```python
from build123d import *

# Parameters (mm, degrees)
BOSS_EXTRUDE2_DEPTH  = 3.81
FILLET1_R            = 3.175
CUT_EXTRUDE1_REACH   = 61.178
SKETCH4_R            = 1.627
FILLET2_R            = 1.27
CUT_EXTRUDE2_REACH   = 60.809
SKETCH5_R            = 1.905
SKETCH6_W            = 38.1
SKETCH6_H            = 11.43
BOSS_EXTRUDE3_DEPTH  = 7.62
SKETCH7_R            = 2.54
BOSS_EXTRUDE4_DEPTH  = 8.89
SKETCH8_R            = 4.445
BOSS_EXTRUDE5_DEPTH  = 2
FILLET3_R            = 1.27
FILLET3_OF_MIRROR3_R = 1.27
FILLET4_R            = 0.635
CUT_EXTRUDE3_START   = -0.508
CUT_EXTRUDE3_DEPTH   = 0.508
SKETCH13_W           = 12.7
SKETCH13_H           = 3.81
CUT_EXTRUDE4_DEPTH   = 1.778
SKETCH14_W           = 11.811
SKETCH14_H           = 2.54
CUT_EXTRUDE5_DEPTH   = 2.54
SKETCH15_W           = 15.24
SKETCH15_H           = 6.35
BOSS_EXTRUDE6_DEPTH  = 1.778
BOSS_EXTRUDE7_DEPTH  = 2.54
BOSS_EXTRUDE8_DEPTH  = 2.54


# Read off the part's stored shape, not the designer's step: Cut-Extrude3
with BuildPart() as part:
    # Sketch3 → Boss-Extrude2 (new, symmetric)
    with BuildSketch(Plane.XY):
        Polygon((34.29, -3.175), (34.29, 3.175), (26.67, 3.175), (26.67, 41.275), (34.29, 41.275), (34.29, 47.625), (0, 47.625), (-34.29, 47.625), (-34.29, 41.275), (-26.67, 41.275), (-26.67, 3.175), (-34.29, 3.175), (-34.29, -3.175), (-19.05, -3.175), (-19.05, 0), (19.05, 0), (19.05, -3.175), align=None)
        Polygon((-19.05, 3.175), (-19.05, 41.275), (0, 41.275), (19.05, 41.275), (19.05, 3.175), align=None, mode=Mode.SUBTRACT)
    extrude(amount=BOSS_EXTRUDE2_DEPTH, both=True)

    # Fillet1
    fillet1_edges = [part.edges().sort_by_distance(p)[0] for p in [
        (34.29, 3.175, 0),
        (34.29, 41.275, 0),
        (34.29, 47.625, 0),
        (-34.29, 3.175, 0),
        (-34.29, 41.275, 0),
        (-34.29, 47.625, 0),
        (34.29, -3.175, 0),
        (-34.29, -3.175, 0),
    ]]
    fillet(fillet1_edges, radius=FILLET1_R - 0.0001)  # a hair under: the kernel refuses the full size

    # Sketch4 → Cut-Extrude1 (cut, up to next)
    with BuildSketch(Plane.XY.offset(3.81), mode=Mode.PRIVATE) as cut_extrude1_sk1:
        with Locations((-31.115, 44.45)):
            Circle(SKETCH4_R)
    cut_extrude1_tool1 = extrude(cut_extrude1_sk1.sketch, amount=-CUT_EXTRUDE1_REACH, mode=Mode.PRIVATE) & part.part
    # Sketch4 → Cut-Extrude1 (cut, up to next)
    with BuildSketch(Plane.XY.offset(3.81), mode=Mode.PRIVATE) as cut_extrude1_sk2:
        with Locations((-31.115, 0)):
            Circle(SKETCH4_R)
    cut_extrude1_tool2 = extrude(cut_extrude1_sk2.sketch, amount=-CUT_EXTRUDE1_REACH, mode=Mode.PRIVATE) & part.part
    cut_extrude1_1 = cut_extrude1_tool1.solids().sort_by_distance((-31.115, 44.45, 3.81))[0]
    add(cut_extrude1_1, mode=Mode.SUBTRACT)
    cut_extrude1_2 = cut_extrude1_tool2.solids().sort_by_distance((-31.115, 0, 3.81))[0]
    add(cut_extrude1_2, mode=Mode.SUBTRACT)
    cut_extrude1 = cut_extrude1_1 + cut_extrude1_2  # Cut-Extrude1 as one shape, for the pattern or mirror that repeats it

    # Mirror1: Cut-Extrude1 across plane
    add(cut_extrude1.mirror(Plane(origin=(0, 0, 0), x_dir=(0, 0, 1), z_dir=(1, 0, 0))), mode=Mode.SUBTRACT)

    # Fillet2
    fillet2_edges = [part.edges().sort_by_distance(p)[0] for p in [
        (-26.67, 22.225, -3.81),
        (26.67, 22.225, -3.81),
        (26.67, 22.225, 3.81),
        (-26.67, 22.225, 3.81),
    ]]
    fillet(fillet2_edges, radius=FILLET2_R)

    # Sketch5 → Cut-Extrude2 (cut, up to next)
    with BuildSketch(Plane.XZ, mode=Mode.PRIVATE) as cut_extrude2_sk1:
        with Locations((-15.24, 0)):
            Circle(SKETCH5_R)
    cut_extrude2_tool1 = extrude(cut_extrude2_sk1.sketch, amount=-CUT_EXTRUDE2_REACH, mode=Mode.PRIVATE) & part.part
    # Sketch5 → Cut-Extrude2 (cut, up to next)
    with BuildSketch(Plane.XZ, mode=Mode.PRIVATE) as cut_extrude2_sk2:
        with Locations(Location((15.24, 0, 0), (0, 0, 180))):
            Circle(SKETCH5_R)
    cut_extrude2_tool2 = extrude(cut_extrude2_sk2.sketch, amount=-CUT_EXTRUDE2_REACH, mode=Mode.PRIVATE) & part.part
    add(cut_extrude2_tool1.solids().sort_by_distance((-15.24, 0, 0))[0], mode=Mode.SUBTRACT)
    add(cut_extrude2_tool2.solids().sort_by_distance((15.24, 0, 0))[0], mode=Mode.SUBTRACT)

    # Sketch6 → Boss-Extrude3 (add)
    with BuildSketch(Plane.XY.offset(3.81)):
        with Locations((0, 11.1125)):
            Rectangle(SKETCH6_W, SKETCH6_H)
    extrude(amount=-BOSS_EXTRUDE3_DEPTH)

    # Sketch7 → Boss-Extrude4 (add)
    with BuildSketch(Plane.XY.offset(3.81)):
        with Locations(Location((-8.89, 11.176999998, 0), (0, 0, 180))):
            Circle(SKETCH7_R)
        with Locations(Location((8.89, 11.176999998, 0), (0, 0, 180))):
            Circle(SKETCH7_R)
    extrude(amount=BOSS_EXTRUDE4_DEPTH)

    # Sketch8 → Boss-Extrude5 (add)
    with BuildSketch(Plane.XY.offset(3.81)):
        with Locations(Location((-8.89, 11.176999998, 0), (0, 0, 180))):
            Circle(SKETCH8_R)
    boss_extrude5 = extrude(amount=BOSS_EXTRUDE5_DEPTH)

    # Fillet3
    fillet3_edges = [part.edges().sort_by_distance(p)[0] for p in [
        (-4.445, 11.176999998, 5.81),
    ]]
    fillet(fillet3_edges, radius=FILLET3_R)

    # Mirror3: Boss-Extrude5 across plane
    add(boss_extrude5.mirror(Plane(origin=(0, 0, 0), x_dir=(0, 0, 1), z_dir=(1, 0, 0))))

    # Fillet3 of Mirror3
    fillet3_of_mirror3_edges = [part.edges().sort_by_distance(p)[0] for p in [
        (4.445, 11.176999998, 5.81),
    ]]
    fillet(fillet3_of_mirror3_edges, radius=FILLET3_OF_MIRROR3_R)

    # Fillet4
    fillet4_edges = [part.edges().sort_by_distance(p)[0] for p in [
        (19.05, 4.28625, 3.81),
        (19.05, 4.28625, -3.81),
        (-19.05, 4.28625, 3.81),
        (-19.05, 4.28625, -3.81),
        (0, 16.8275, 3.81),
        (19.05, 3.175, 0),
        (-19.05, 3.175, 0),
        (0, 3.175, -3.81),
        (0, 3.175, 3.81),
    ]]
    fillet(fillet4_edges, radius=FILLET4_R)

    # Cut-Extrude3 outline → Cut-Extrude3 (cut)
    with BuildSketch(Plane(origin=(0, 0, -3.81), x_dir=(-1, 0, 0), z_dir=(0, 0, -1)).offset(CUT_EXTRUDE3_START)):
        Polygon((-36, 41.275), (-25.4, 41.275), (-25.4, 3.175), (-36, 3.175), (-36, -5), (36, -5), (36, 3.175), (25.4, 3.175), (25.4, 41.275), (36, 41.275), (36, 49), (-36, 49), align=None)
    extrude(amount=CUT_EXTRUDE3_DEPTH, mode=Mode.SUBTRACT)

    # Sketch13 → Cut-Extrude4 (cut)
    with BuildSketch(Plane.XY.offset(3.81)):
        with Locations((0, 43.18)):
            Rectangle(SKETCH13_W, SKETCH13_H)
    extrude(amount=-CUT_EXTRUDE4_DEPTH, mode=Mode.SUBTRACT)

    # Sketch14 → Cut-Extrude5 (cut)
    with BuildSketch(Plane(origin=(0, 0, -3.302), x_dir=(-1, 0, 0), z_dir=(0, 0, -1))):
        with Locations((0, 15.5575)):
            Rectangle(SKETCH14_W, SKETCH14_H)
    extrude(amount=-CUT_EXTRUDE5_DEPTH, mode=Mode.SUBTRACT)

    # Sketch15 → Boss-Extrude6 (add)
    with BuildSketch(Plane(origin=(0, 0, -3.302), x_dir=(-1, 0, 0), z_dir=(0, 0, -1))):
        with Locations((0, 44.45)):
            Rectangle(SKETCH15_W, SKETCH15_H)
        Polygon((-7.62, 16.8275), (-5.9055, 16.8275), (-5.9055, 14.2875), (5.9055, 14.2875), (5.9055, 16.8275), (7.62, 16.8275), (7.62, 9.2075), (-7.62, 9.2075), align=None)
    extrude(amount=BOSS_EXTRUDE6_DEPTH)

    # Sketch16 → Boss-Extrude7 (add)
    with BuildSketch(Plane(origin=(0, 0, -5.08), x_dir=(-1, 0, 0), z_dir=(0, 0, -1))):
        Polygon((-5.9055, 41.275), (-5.9055, 42.926), (5.9055, 42.926), (5.9055, 41.275), (7.62, 41.275), (7.62, 47.625), (-7.62, 47.625), (-7.62, 41.275), align=None)
    extrude(amount=BOSS_EXTRUDE7_DEPTH)

    # Sketch18 → Boss-Extrude8 (add)
    with BuildSketch(Plane(origin=(0, 0, -5.08), x_dir=(-1, 0, 0), z_dir=(0, 0, -1))):
        Polygon((-7.62, 16.8275), (-5.9055, 16.8275), (-5.9055, 10.4902), (5.9055, 10.4902), (5.9055, 16.8275), (7.62, 16.8275), (7.62, 9.2075), (-7.62, 9.2075), align=None)
    extrude(amount=BOSS_EXTRUDE8_DEPTH)


solid = part.part
```
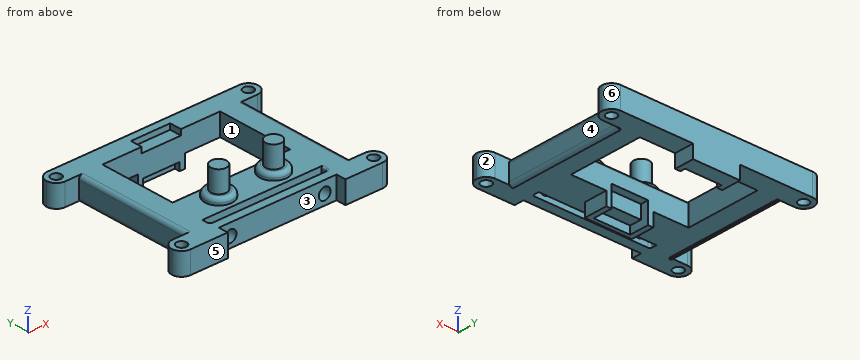
Source: CAD feature listing. Evaluate the final solid. Frame: model axes, mm. Face numbers are marked on the shaded views. A direction names the side the tool comes from. Coordinates: 2 decimals unless noted, no trailing zeros. Order: outer loops, then holes, each group sorted by start corner. A loop starts at its lowest first (then second) coordinate and runs counter-clockwise, first axis right, second up. Notation, with made-up numbers: (-6, 33.5) - (12, 33.5) arc R20 cw to (12, 42.5) - close; hole circle Ø10 at (-25.5, -38.5). An arc over 180 degrees is marked (long way). One line per item, written item: value.
1) Mould query, pull axis Y, two halves, no side actions, for the marked faces 4, 5 and 6. Classes: released by +Y, released by -Y, zero draft, split by the parting line, or undercut.
Computed values:
face 4: undercut
face 5: released by -Y
face 6: released by +Y
2) Cut plane B-B on y = 30.5. Output: boundary loops of the cut face in (x, z).
Computed values:
outline: (-26.67, -2.54) arc R1.27 ccw to (-25.4, -3.81) - (-25.4, -3.3) - (-19.05, -3.3) - (-19.05, 3.81) - (-25.4, 3.81) arc R1.27 ccw to (-26.67, 2.54) - close; (19.05, -3.3) - (25.4, -3.3) - (25.4, -3.81) arc R1.27 ccw to (26.67, -2.54) - (26.67, 2.54) arc R1.27 ccw to (25.4, 3.81) - (19.05, 3.81) - close
3) Reachability of the marked faces 1, 2 and 3 from +Z, -Z, +X, -X, +Y, -Y: full face, straight path, thin tool, end or side. Return the list, or none.
Computed values:
face 1: +Z, -Z
face 2: +Z, -Z, +X
face 3: +Z, -Z, -Y
4) Contact query for flat-ended pins moving along their axis: pin 1 (3.5 mm diameter, centred on y = -2, z = -0.5, fed in from +X); pin 2 (4.5 mm diameter, centred on x = 15.24, z = 0, fed in from -Y); pin 3 (4.5 mm diameter, centred on x = 3.5, z = -6, fed in from -Y). Output: stop coordinate, or through.
Computed values:
pin 1: stops at x = 34.28
pin 2: stops at y = 0
pin 3: stops at y = 9.21
5) Ray query, line 1 (Y direction, x = -6.5, z = 0.25) (1 decimal); line 2 (Y direction, x = 1, z = -1.75) (1 decimal); line 3 (Y direction, x = -26.5, z = 3.5) (3 decimals). Return the intervals inside material, ascending. Write a range as [from, to].
Computed values:
line 1: y = [0, 3.2], [5.4, 16.8], [41.3, 47.6]
line 2: y = [0, 3.2], [5.4, 14.3], [41.3, 47.6]
line 3: y = [-3.175, 3.175], [41.275, 47.625]
6) Cut plane A-A on x = -0.5. State how many separate pieces and enclosed holes the cut face has, plus the area to 3 significant figures.
Computed values:
separate pieces: 3
enclosed holes: 0
area: 171 mm^2
